from build123d import *

# Parameters (mm, degrees)
SKETCH1_R           = 9.475
BOSS_EXTRUDE1_DEPTH = 12.35
SKETCH2_R           = 2.445
CUT_EXTRUDE1_DEPTH  = 10
SKETCH3_R           = 3.925
CUT_EXTRUDE2_DEPTH  = 19


with BuildPart() as part:
    # Sketch1 → Boss-Extrude1 (new, symmetric)
    with BuildSketch(Plane(origin=(0, 0, 0), x_dir=(1, 0, 0), z_dir=(0, 1, 0))):
        with Locations(Location((0, 0, 0), (0, 0, 270))):
            Circle(SKETCH1_R)
    extrude(amount=BOSS_EXTRUDE1_DEPTH, both=True)

    # Sketch2 → Cut-Extrude1 (cut)
    with BuildSketch(Plane(origin=(0, 12.35, 0), x_dir=(1, 0, 0), z_dir=(0, 1, 0))):
        with Locations(Location((0, 0, 0), (0, 0, 270))):
            Circle(SKETCH2_R)
    extrude(amount=-CUT_EXTRUDE1_DEPTH, mode=Mode.SUBTRACT)

    # Sketch3 → Cut-Extrude2 (cut)
    with BuildSketch(Plane.XZ.offset(12.35)):
        with Locations(Location((0, 0, 0), (0, 0, 270))):
            Circle(SKETCH3_R)
    extrude(amount=-CUT_EXTRUDE2_DEPTH, mode=Mode.SUBTRACT)


solid = part.part
Model file for the job. Use its own axes, mm. A direction names the side the tool comes from. Give positions to 0.01 mm unless a question says otherwise; leave off trailing zeros. Order: outer loops, then holes, each group sorted by start corner. A loop starts at its lowest first (then second) coordinate and runs counter-clockwise, first axis right, second up. Notation, with made-up numbers: (-35.5, 39) - (-15.5, 39) arc R13 cw to (-15.5, 58) - close; hole circle Ø5 at (47.25, 79). An arc over 180 degrees is marked (long way). Return JSON: item names as keys, results as strings.
1) Flat gauge pins, fed straight in: P1, Ø8, axis at y = 9, z = -4, coming from the -X side (3 decimals); P2, Ø10, axis at y = -0.5, z = 6, coming from the -X side; P3, Ø1, axis at x = -3, y = -2, coming from the -Z side; P4, Ø10, axis at x = 6.5, y = -4.5, coming from the -Z side. Where does each tip first touch, or does it go through?
Geometry says:
{"P1": "x = -9.475", "P2": "x = -9.42", "P3": "z = -9.14", "P4": "z = -9.36"}
2) Cut at D-D, the plane x = -3.5. Give the cut face in (y, z).
Geometry says:
{"outline": "(-12.35, -8.8) - (12.35, -8.8) - (12.35, 8.8) - (-12.35, 8.8) - (-12.35, 1.78) - (6.65, 1.78) - (6.65, -1.78) - (-12.35, -1.78) - close"}
3) Cut at C-C, the plane y = -6. Give the cut face in (x, z) (3 decimals).
Geometry says:
{"outline": "circle Ø18.95 at (0, 0); hole circle Ø7.85 at (0, 0)"}
4) 3-axis set-ups, long thin cutter, end or side, ignore diameter. For faces 1 (the cylindrical face through (-2.388, -2.983, 3.115)), 2 (the cylindrical face through (-1.49, 9.54, -1.94)): which of +Z, -Z, +X, -X, +Y, -Y reach the whole face in a straight line?
Geometry says:
{"face 1": "-Y", "face 2": "+Y, -Y"}
5) Cut at B-B, the plane z = 0. Give the cut face in (x, y) (3 decimals), plus the area to 3 significant figures.
Geometry says:
{"outline": "(-9.475, -12.35) - (-3.925, -12.35) - (-3.925, 6.65) - (-2.445, 6.65) - (-2.445, 12.35) - (-9.475, 12.35) - close; (2.445, 6.65) - (3.925, 6.65) - (3.925, -12.35) - (9.475, -12.35) - (9.475, 12.35) - (2.445, 12.35) - close", "area": "291 mm²"}
6) Pull direction Z, two halves, no side cores. Call faces 3 (the cylindrical face through (-9.25, 0.17, -2.05)), 4 (the flat face through (0.1, -12.35, 4.1)), 5 (the flat face through (-2, 6.65, 2)): pulls with the +Z half, pulls with the -Z half, needs draft (parallel to the pull), parting line crosses it, or undercut.
Geometry says:
{"face 3": "parting line crosses it", "face 4": "needs draft", "face 5": "undercut"}
7) Probe line 1 (X direction, y = 1.5, z = 0) (3 decimals); line 2 (X direction, y = 9.9, z = 0) (3 decimals); line 3 (Z direction, x = 0.25, y = 5.75). List the from-to ranges inside material, lowest first. Write a range as from..to.
Geometry says:
{"line 1": "-9.475..-3.925, 3.925..9.475", "line 2": "-9.475..-2.445, 2.445..9.475", "line 3": "-9.47..-3.92, 3.92..9.47"}
8) Cut at A-A, the plane x = 0. Give the cut face in (y, z) (3 decimals).
Geometry says:
{"outline": "(-12.35, -9.475) - (12.35, -9.475) - (12.35, -2.445) - (6.65, -2.445) - (6.65, -3.925) - (-12.35, -3.925) - close; (-12.35, 3.925) - (6.65, 3.925) - (6.65, 2.445) - (12.35, 2.445) - (12.35, 9.475) - (-12.35, 9.475) - close"}
